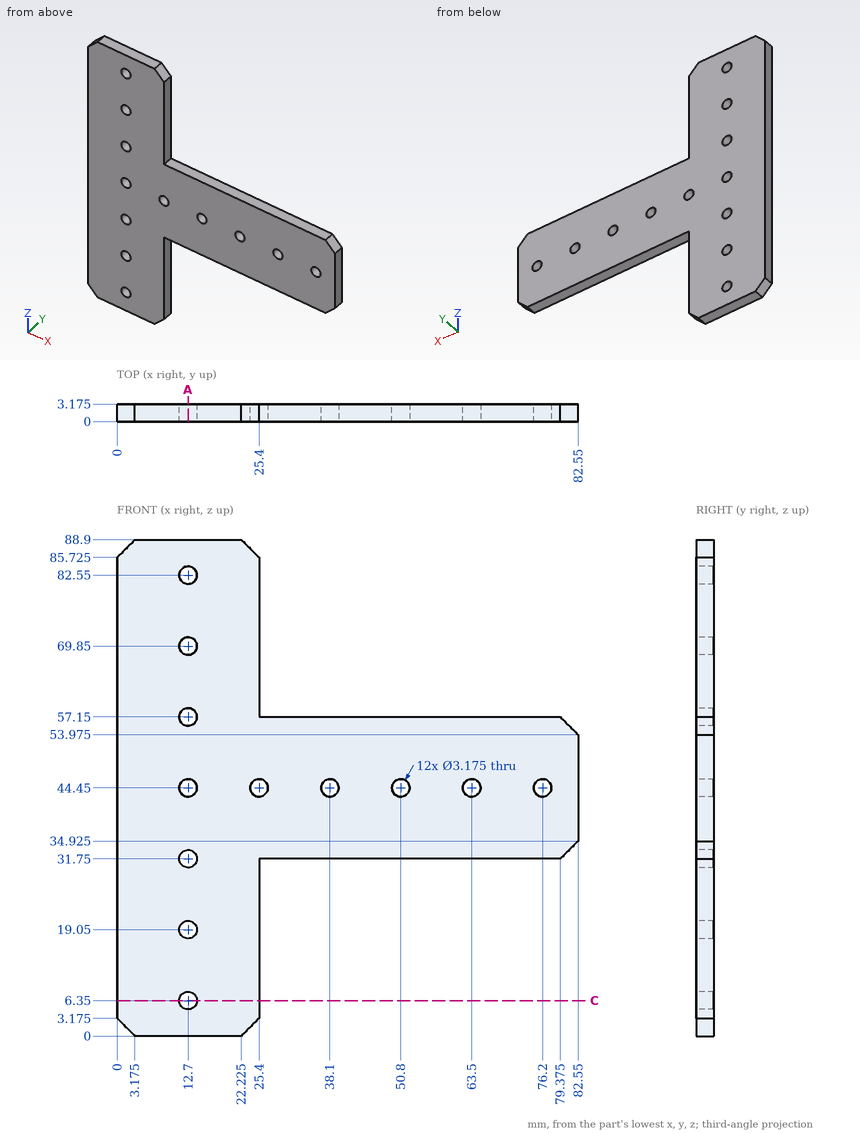
Answer from the drawing. Dimensions are ordinates in mm from the lowest x, y and z of the part. Round coordinates to 2 decimals unless told otherwise and drop trailing zeros. Write each loop counter-clockwise with the first axis right and the second up, starting at its lowest first coordinate (ties: lowest second). Pieces come first, ordered by that corner, then holes.
1. The part is cut by section C-C, the plane z = 6.35. Determine the outline of the cut face in (x, y) (1 decimal).
2. Given pin 1 Ø1.6 at (y, z) = (2, 67.5) entering from +X; pin 2 Ø5 at (x, z) = (28.5, 68.5) entering from -Y; pin 3 Ø1.6 at (x, y) = (50.5, 2) entering from -Z, each flat-ended and moving along its own axis, determine where each tip first touches the part or whether it passes through.
3. The part is cut by section A-A, the plane x = 12.7. State how many separate pieces and enclosed holes the cut face has, then the cut area to 3 significant figures.
4. Straight lines are drawn through the part: L1, parallel to Z at x = 76.2, y = 0.7; L2, parallel to X at y = 0.1, z = 56 (3 decimals); L3, parallel to X at y = 0.2, z = 21.5. For each, find the intervals that lie inside material, in ascending order.
Values:
1. outline: (0, 0) - (11.1, 0) - (11.1, 3.2) - (0, 3.2) - close; (14.3, 0) - (25.4, 0) - (25.4, 3.2) - (14.3, 3.2) - close
2. pin 1: stops at x = 25.4
2. pin 2: passes through
2. pin 3: stops at z = 31.75
3. separate pieces: 8
3. enclosed holes: 0
3. area: 212 mm2
4. L1: z = 31.75 to 42.86, 46.04 to 57.15
4. L2: x = 0 to 11.606, 13.794 to 80.525
4. L3: x = 0 to 25.4
